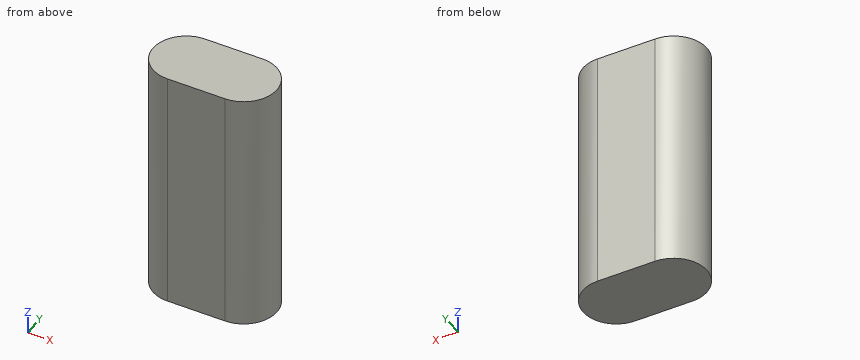
from build123d import *

# Parameters (mm, degrees)
SKETCH1_W           = 37.5
SKETCH1_H           = 74
BOSS_EXTRUDE1_DEPTH = 20
FILLET3_RADIUS      = 10
FILLET3_LENGTH      = 74
FILLET4_RADIUS      = 10
FILLET4_LENGTH      = 74


with BuildPart() as part:
    # Sketch1 → Boss-Extrude1 (new body)
    with BuildSketch(Plane(origin=(0, 0, 0), x_dir=(1, 0, 0), z_dir=(0, 1, 0))):
        Rectangle(SKETCH1_W, SKETCH1_H)
    extrude(amount=BOSS_EXTRUDE1_DEPTH)

    # Fillet3: full round fillet: the end face becomes a half cylinder, R = half its width
    fillet3_face = Plane((-18.75, 10, 0), x_dir=(0, 0, -1), z_dir=(-1, 0, 0))  # on the end face: x along it, z out of the body
    fillet3_slab = fillet3_face.offset(-FILLET3_RADIUS / 2) * Box(FILLET3_LENGTH, 2 * FILLET3_RADIUS, FILLET3_RADIUS, mode=Mode.PRIVATE)  # the body's end, R deep
    fillet3_round = Plane((-8.75, 10, 0), x_dir=(-1, 0, 0), z_dir=(0, 0, -1)) * Cylinder(FILLET3_RADIUS, FILLET3_LENGTH, mode=Mode.PRIVATE)  # its axis R under the face
    add(fillet3_slab - fillet3_round, mode=Mode.SUBTRACT)

    # Fillet4: full round fillet: the end face becomes a half cylinder, R = half its width
    fillet4_face = Plane((18.75, 10, 0), x_dir=(0, 0, 1), z_dir=(1, 0, 0))  # on the end face: x along it, z out of the body
    fillet4_slab = fillet4_face.offset(-FILLET4_RADIUS / 2) * Box(FILLET4_LENGTH, 2 * FILLET4_RADIUS, FILLET4_RADIUS, mode=Mode.PRIVATE)  # the body's end, R deep
    fillet4_round = Plane((8.75, 10, 0), x_dir=(1, 0, 0), z_dir=(0, 0, 1)) * Cylinder(FILLET4_RADIUS, FILLET4_LENGTH, mode=Mode.PRIVATE)  # its axis R under the face
    add(fillet4_slab - fillet4_round, mode=Mode.SUBTRACT)


solid = part.part
The model under review builds one solid part; all positions refer to its coordinate system, in mm. Round coordinates to 2 decimals unless told otherwise and drop trailing zeros. Loops run counter-clockwise (first coordinate to the right, second up) from the corner with the lowest first, then second, coordinate; pieces in that order, holes last. Notation, with made-up numbers: (27, -20.5) -> (59, -20.5) arc R16 cw to (59, 7.5) -> close; hole circle Ø4 at (5.25, 16). An arc over 180 degrees is marked (long way). One line per question, with ' | ' between items. Start each with the question number.
Item 1: Add section B-B, the plane z = -31. Write out the cut boundary in (x, y), then the cut area to 3 significant figures.
Item 2: Wall thickness on line 1 along X through (y, z) = (1.5, -26.5); line 2 along Y through (x, z) = (-15.5, -28); line 3 along Y through (x, z) = (15, -6.5): over which ranges is each line inside the solid? List them lowest first. Write a range as [from, to].
Item 3: Add section A-A, the plane y = 18. Write out the cut boundary in (x, z), then the cut area to 3 significant figures.
Item 4: For pin 1 (1 mm diameter, centred on x = 9.5, z = 21.5, fed in from -Y); pin 2 (3 mm diameter, centred on y = 2, z = -4.5, fed in from +X); pin 3 (4 mm diameter, centred on y = 3.5, z = -27, fed in from +X), all flat-tipped, find the tip position at first contact; note any pin that passes through.
Return value:
1) outline: (-8.75, 0) -> (8.75, 0) arc R10 ccw to (8.75, 20) -> (-8.75, 20) arc R10 ccw to start | area: 664 mm2
2) line 1: x = [-14.02, 14.02] | line 2: y = [2.62, 17.38] | line 3: y = [2.19, 17.81]
3) outline: (-14.75, -37) -> (14.75, -37) -> (14.75, 37) -> (-14.75, 37) -> close | area: 2,180 mm2
4) pin 1: stops at y = 0 | pin 2: stops at x = 16.35 | pin 3: stops at x = 17.68
